The listing builds one solid part. Answer for the finished solid, in the listing's coordinates (mm). Face numbers are marked on the shaded views. Give positions to 0.01 mm unless a question says otherwise; leave off trailing zeros. Order: outer loops, then holes, each group sorted by start corner. A loop starts at its lowest first (then second) coordinate and runs counter-clockwise, first axis right, second up. Notation, with made-up numbers: (69, 3) -> (80, 3) arc R13 ccw to (80, 26) -> close; hole circle Ø2 at (80, -33.5). An arc over 180 degrees is marked (long way). One line per question, with ' | ' between items. Start each with the question number.
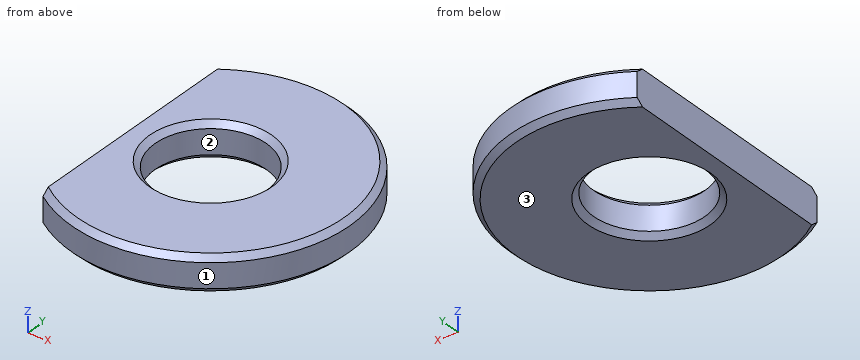
```python
from build123d import *

# Parameters (mm, degrees)
SKETCH_2_W          = 25
SKETCH_2_H          = 25
CUT_EXTRUDE_1_DEPTH = 3.2


with BuildPart() as part:
    # Sketch 1 → Revolve 1 (revolve)
    with BuildSketch(Plane(origin=(0, 0, 0), x_dir=(1, 0, 0), z_dir=(0, 1, 0)), mode=Mode.PRIVATE) as revolve_1_sk:
        Polygon((5, 2.7), (5, 0.5), (5.5, 0), (12, 0), (12.5, 0.5), (12.5, 2.7), (12, 3.2), (5.5, 3.2), align=None)
    revolve(revolve_1_sk.sketch.rotate(Axis((0, 0, 3), (0, 0, -1)), 180), axis=Axis((0, 0, 3), (0, 0, -1)))

    # Sketch 2 → Cut-Extrude 1 (cut)
    with BuildSketch(Plane.XY):
        with Locations((-19.5, 0)):
            Rectangle(SKETCH_2_W, SKETCH_2_H)
    extrude(amount=-CUT_EXTRUDE_1_DEPTH, mode=Mode.SUBTRACT)


solid = part.part
```
(1) Determine the mould class of the marked faces 1, 2 and 3 for opening direction X: pulls with the +X half, pulls with the -X half, needs draft (parallel to the pull), parting line crosses it, or undercut.
(2) Given P1, Ø1, axis at x = -2.5, z = -2, coming from the -Y side; P2, Ø5, axis at x = -2.5, y = -0.5, coming from the -Z side, each flat-ended and moving along its own axis, determine where each tip first touches the part or whether it passes through.
(3) The part is cut by section A-A on y = 0. Determine the outline of the cut face in (x, z), plus the area to 4 significant figures.
(4) The part is cut by section B-B on x = 0. Determine the outline of the cut face in (y, z).
(5) Consider line 1 (Y direction, x = 0, z = -1); line 2 (X direction, y = 1.5, z = -2.65); line 3 (X direction, y = -1, z = -0.8). Determine where each line is inside the solid, lowest interval first.
(6) The part is cut by section C-C on z = -2.2. Determine the outline of the cut face in (x, y).
Result sheet:
1) face 1: parting line crosses it | face 2: undercut | face 3: needs draft
2) P1: stops at y = -12.34 | P2: stops at z = -2.75
3) outline: (-7, -3.2) -> (-5.5, -3.2) -> (-5, -2.7) -> (-5, -0.5) -> (-5.5, 0) -> (-7, 0) -> close; (5, -2.7) -> (5.5, -3.2) -> (12, -3.2) -> (12.5, -2.7) -> (12.5, -0.5) -> (12, 0) -> (5.5, 0) -> (5, -0.5) -> close | area: 29.65 mm^2
4) outline: (-12.5, -2.7) -> (-12, -3.2) -> (-5.5, -3.2) -> (-5, -2.7) -> (-5, -0.5) -> (-5.5, 0) -> (-12, 0) -> (-12.5, -0.5) -> close; (5, -2.7) -> (5.5, -3.2) -> (12, -3.2) -> (12.5, -2.7) -> (12.5, -0.5) -> (12, 0) -> (5.5, 0) -> (5, -0.5) -> close
5) line 1: y = -12.5 to -5, 5 to 12.5 | line 2: x = -7 to -4.77, 4.77 to 12.41 | line 3: x = -7 to -4.9, 4.9 to 12.46
6) outline: (-7, -10.36) arc R12.5 ccw (long way) to (-7, 10.36) -> close; hole circle Ø10 at (0, 0)
